from build123d import *

# Parameters (mm, degrees)
BOSS_EXTRUDE1_DEPTH = 2.5
SKETCH2_R           = 1.2
CUT_EXTRUDE1_DEPTH  = 8
FILLET1_R           = 1.5


with BuildPart() as part:
    # Sketch1 → Boss-Extrude1 (new body, symmetric)
    with BuildSketch(Plane.XY):
        with BuildLine():
            Line((5.5, 0), (12.7, 0))
            Line((12.7, 0), (12.7, -1.5))
            Line((12.7, -1.5), (6.837397166, -1.5))
            ThreePointArc((6.837397166, -1.5), (0, -7), (-6.837397166, -1.5))
            Line((-6.837397166, -1.5), (-12.7, -1.5))
            Line((-12.7, -1.5), (-12.7, 0))
            Line((-12.7, 0), (-5.5, 0))
            ThreePointArc((-5.5, 0), (0, -5.5), (5.5, 0))
        make_face()
    extrude(amount=BOSS_EXTRUDE1_DEPTH, both=True)

    # Sketch2 → Cut-Extrude1 (cut, through all)
    with BuildSketch(Plane(origin=(0, 0, 0), x_dir=(1, 0, 0), z_dir=(0, 1, 0))):
        with Locations((-10.2, 0)):
            Circle(SKETCH2_R)
        with Locations((10.2, 0)):
            Circle(SKETCH2_R)
    extrude(amount=-CUT_EXTRUDE1_DEPTH, mode=Mode.SUBTRACT)

    # Fillet1
    fillet1_edges = [part.edges().sort_by_distance(p)[0] for p in [
        (6.837397166, -1.5, 0),
        (-6.837397166, -1.5, 0),
    ]]
    fillet(fillet1_edges, radius=FILLET1_R)


solid = part.part
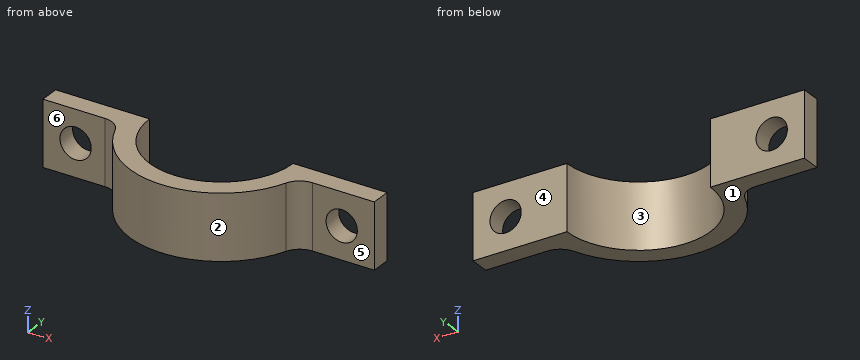
The model under review builds one solid part; all positions refer to its coordinate system, in mm. Face numbers are marked on the shaded views. A direction names the side the tool comes from. Coordinates: 2 decimals unless noted, no trailing zeros. Order: outer loops, then holes, each group sorted by start corner. A loop starts at its lowest first (then second) coordinate and runs counter-clockwise, first axis right, second up. Notation, with made-up numbers: (-27, 2.5) -> (-3, 2.5) arc R31 cw to (-3, 26.5) -> close; hole circle Ø2 at (26.5, -30.5). An arc over 180 degrees is marked (long way). Answer in a Markdown table with one row per item.
(1) The part is to be moulded in two halves that separate along X. For the marked faces 1, 2 and 3, say which applies: +X half, -X half, draft (parallel to the pull), parting line (faces both ways), or undercut.
Answers:
| item | result |
|---|---|
| face 1 | draft |
| face 2 | parting line |
| face 3 | undercut |
(2) Insertion check: pin 1 (2 mm diameter, centred on x = -7, z = 1, fed in from -Y); pin 2 (1.4 mm diameter, centred on x = 11, z = -1, fed in from -Y); pin 3 (1.9 mm diameter, centred on x = -10.2, z = 0, fed in from -Y); pin 4 (1.5 mm diameter, centred on x = 3, z = -1.5, fed in from +Y). Each pin has a flat end and moves straight along its axis. Give the tip position at first contact, or say it passes through.
Answers:
| item | result |
|---|---|
| pin 1 | y = -3.61 |
| pin 2 | y = -1.5 |
| pin 3 | through |
| pin 4 | y = -4.02 |
(3) Consider section B-B (x = -10.2). Write out the cut boundary in (y, z).
Answers:
| item | result |
|---|---|
| outline | (-1.5, -2.5) -> (0, -2.5) -> (0, -1.2) -> (-1.5, -1.2) -> close; (-1.5, 1.2) -> (0, 1.2) -> (0, 2.5) -> (-1.5, 2.5) -> close |
(4) Consider section C-C (y = -3.75). Write out the cut boundary in (x, z), plus the area to 3 significant figures.
Answers:
| item | result |
|---|---|
| outline | (-5.91, -2.5) -> (-4.02, -2.5) -> (-4.02, 2.5) -> (-5.91, 2.5) -> close; (4.02, -2.5) -> (5.91, -2.5) -> (5.91, 2.5) -> (4.02, 2.5) -> close |
| area | 18.9 mm² |
(5) Machinability: for the marked faces 4, 5 and 6, which of the approach directions +Z, -Z, +X, -X, +Y, -Y give a long, thin tool a straight path to every point of the face, cutting with its end or side? Answer none if there is none.
Answers:
| item | result |
|---|---|
| face 4 | +Z, -Z, +X, -X, +Y |
| face 5 | +Z, -Z, +X, -Y |
| face 6 | +Z, -Z, -X, -Y |
(6) Wall thickness on line 1 along Z through (x, y) = (10.2, -0.35); line 2 along X through (y, z) = (-0.4, 0); line 3 along X through (y, z) = (-0.25, 0.95): over which ranges is each line inside the solid? List them lowest first.
Answers:
| item | result |
|---|---|
| line 1 | -2.5 to -1.2, 1.2 to 2.5 |
| line 2 | -12.7 to -11.4, -9 to -5.49, 5.49 to 9, 11.4 to 12.7 |
| line 3 | -12.7 to -10.93, -9.47 to -5.49, 5.49 to 9.47, 10.93 to 12.7 |
(7) Consider section A-A (z = 0). Write out the cut boundary in (x, y), plus the area to 3 significant figures.
Answers:
| item | result |
|---|---|
| outline | (-12.7, -1.5) -> (-11.4, -1.5) -> (-11.4, 0) -> (-12.7, 0) -> close; (-9, -1.5) -> (-7.95, -1.5) arc R1.5 cw to (-6.55, -2.47) arc R7 ccw to (6.55, -2.47) arc R1.5 cw to (7.95, -1.5) -> (9, -1.5) -> (9, 0) -> (5.5, 0) arc R5.5 cw to (-5.5, 0) -> (-9, 0) -> close; (11.4, -1.5) -> (12.7, -1.5) -> (12.7, 0) -> (11.4, 0) -> close |
| area | 40.0 mm² |
(8) Consider section D-D (z = -2.05). Write out the cut boundary in (x, y).
Answers:
| item | result |
|---|---|
| outline | (-12.7, -1.5) -> (-7.95, -1.5) arc R1.5 cw to (-6.55, -2.47) arc R7 ccw to (6.55, -2.47) arc R1.5 cw to (7.95, -1.5) -> (12.7, -1.5) -> (12.7, 0) -> (5.5, 0) arc R5.5 cw to (-5.5, 0) -> (-12.7, 0) -> close |
